from build123d import *

# Parameters (mm, degrees)
SKETCH1_R           = 2.4
SKETCH1_R_2         = 1.5
BOSS_EXTRUDE1_DEPTH = 5
FILLET1_R           = 4
FILLET2_R           = 2


with BuildPart() as part:
    # Sketch1 → Boss-Extrude1 (new body)
    with BuildSketch(Plane.XY):
        Polygon((-50, -60), (50, -60), (50, 8), (45.5, 8), (45.5, 36), (50, 36), (50, 60), (29, 60), (29, 39), (-29, 39), (-29, 60), (-50, 60), align=None)
        with Locations((-30, -50)):
            Circle(SKETCH1_R, mode=Mode.SUBTRACT)
        with Locations((30, -50)):
            Circle(SKETCH1_R, mode=Mode.SUBTRACT)
        with Locations((-44, 54)):
            Circle(SKETCH1_R_2, mode=Mode.SUBTRACT)
        with Locations((44, 54)):
            Circle(SKETCH1_R_2, mode=Mode.SUBTRACT)
        with Locations((-44, -11)):
            Circle(SKETCH1_R_2, mode=Mode.SUBTRACT)
        with Locations((44, -11)):
            Circle(SKETCH1_R_2, mode=Mode.SUBTRACT)
    extrude(amount=BOSS_EXTRUDE1_DEPTH)

    # Fillet1
    fillet1_edges = [part.edges().sort_by_distance(p)[0] for p in [
        (50, -60, 2.5),
        (-50, -60, 2.5),
        (-50, 60, 2.5),
        (-29, 60, 2.5),
        (29, 60, 2.5),
        (50, 60, 2.5),
    ]]
    fillet(fillet1_edges, radius=FILLET1_R)

    # Fillet2
    fillet2_edges = [part.edges().sort_by_distance(p)[0] for p in [
        (50, 36, 2.5),
        (50, 8, 2.5),
        (-29, 39, 2.5),
        (29, 39, 2.5),
    ]]
    fillet(fillet2_edges, radius=FILLET2_R)


solid = part.part
Model file for the job. Use its own axes, mm. A direction names the side the tool comes from. Coordinates: 2 decimals unless noted, no trailing zeros. Write each loop counter-clockwise with the first axis right and the second up, starting at its lowest first coordinate (ties: lowest second). Pieces come first, ordered by that corner, then holes. Notation, with made-up numbers: (-20.5, -26.5) -> (29.5, -26.5) arc R19 cw to (29.5, -19.5) -> close; hole circle Ø6 at (73.5, 84). An arc over 180 degrees is marked (long way). One line per item, written item: value. Start each with the question number.
1) Pull direction X, two halves, no side cores. Call faces 4 (the face through (45.5, 22, 2)), 5 (the face through (-1, -12, 0)), 6 (the face through (42.5, -10.93, 2.46)): +X half, -X half, draft (parallel to the pull), parting line (faces both ways), or undercut.
2) Flat gauge pins, fed straight in: pin 1 Ø1.8 at (x, y) = (44, 54) entering from -Z; pin 2 Ø1.5 at (x, z) = (-10, 2) entering from +Y; pin 3 Ø1.2 at (x, z) = (47, 3.5) entering from -Y. Where does each tip first touch, or does it go through?
3) Probe probe 1 along Y at (x, z) = (44, 3.6); probe 2 along X at (y, z) = (51, 0.5); probe 3 along Y at (x, z) = (5, 2.3). List the from-to ranges inside material, lowest first.
4) Slice it at D-D on z = 3.25. Write the cut outline in (x, y).
5) Slice it at C-C on y = 54. Write the cut outline in (x, z).
6) Which spindle directions (+Z, -Z, +X, -X, +Y, -Y) get a long thin tool onto all of the face, cutting with end or side? Do faces 1 (the face through (-30.203, 58.859, 2.535)), 2 (the face through (50, -25, 2)), 3 (the face through (47, 36, 2)). Say none if no direction does.
7) Slice it at A-A on y = -11. Write the cut outline in (x, z), then the cut area to 3 significant figures.
8) Slice it at B-B on x = -44. Write the cut outline in (y, z), then the cut area to 3 significant figures.
Answers follow:
1. face 4: +X half
1. face 5: draft
1. face 6: undercut
2. pin 1: through
2. pin 2: y = 39
2. pin 3: y = -59.98
3. probe 1: -60 to -12.5, -9.5 to 52.5, 55.5 to 60
3. probe 2: -50 to -29, 29 to 50
3. probe 3: -60 to 39
4. outline: (-50, -56) arc R4 ccw to (-46, -60) -> (46, -60) arc R4 ccw to (50, -56) -> (50, 6) arc R2 ccw to (48, 8) -> (45.5, 8) -> (45.5, 36) -> (48, 36) arc R2 ccw to (50, 38) -> (50, 56) arc R4 ccw to (46, 60) -> (33, 60) arc R4 ccw to (29, 56) -> (29, 41) arc R2 cw to (27, 39) -> (-27, 39) arc R2 cw to (-29, 41) -> (-29, 56) arc R4 ccw to (-33, 60) -> (-46, 60) arc R4 ccw to (-50, 56) -> close; hole circle Ø3 at (-44, -11); hole circle Ø3 at (-44, 54); hole circle Ø4.8 at (-30, -50); hole circle Ø4.8 at (30, -50); hole circle Ø3 at (44, -11); hole circle Ø3 at (44, 54)
5. outline: (-50, 0) -> (-45.5, 0) -> (-45.5, 5) -> (-50, 5) -> close; (-42.5, 0) -> (-29, 0) -> (-29, 5) -> (-42.5, 5) -> close; (29, 0) -> (42.5, 0) -> (42.5, 5) -> (29, 5) -> close; (45.5, 0) -> (50, 0) -> (50, 5) -> (45.5, 5) -> close
6. face 1: +Z, -Z, +Y
6. face 2: +Z, -Z, +X, +Y, -Y
6. face 3: +Z, -Z, +X
7. outline: (-50, 0) -> (-45.5, 0) -> (-45.5, 5) -> (-50, 5) -> close; (-42.5, 0) -> (42.5, 0) -> (42.5, 5) -> (-42.5, 5) -> close; (45.5, 0) -> (50, 0) -> (50, 5) -> (45.5, 5) -> close
7. area: 470 mm2
8. outline: (-60, 0) -> (-12.5, 0) -> (-12.5, 5) -> (-60, 5) -> close; (-9.5, 0) -> (52.5, 0) -> (52.5, 5) -> (-9.5, 5) -> close; (55.5, 0) -> (60, 0) -> (60, 5) -> (55.5, 5) -> close
8. area: 570 mm2
